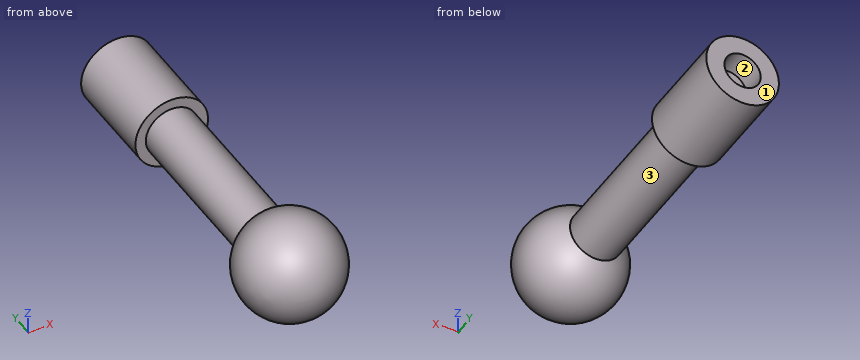
```python
from build123d import *

# Parameters (mm, degrees)
SKETCH3_W          = 7
SKETCH3_H          = 18.520312213
SKETCH4_R          = 3.5
CUT_EXTRUDE1_DEPTH = 5


with BuildPart() as part:
    # Sketch1 → Revolve1 (revolve)
    with BuildSketch(Plane.XY, mode=Mode.PRIVATE) as revolve1_sk:
        with BuildLine():
            Line((0, 41.73429327), (5, 41.73429327))
            Line((5, 41.73429327), (5, -8.26570673))
            ThreePointArc((5, -8.26570673), (9.659258263, -19.514151219), (0, -26.925960768))
            Line((0, -26.925960768), (0, 41.73429327))
        make_face()
    revolve(revolve1_sk.sketch.rotate(Axis((0, 41.73429327, 0), (0, -1, 0)), 180), axis=Axis((0, 41.73429327, 0), (0, -1, 0)))

    # Sketch3 → Revolve3 (revolve)
    with BuildSketch(Plane.XY, mode=Mode.PRIVATE) as revolve3_sk:
        with Locations((3.5, 32.474137164)):
            Rectangle(SKETCH3_W, SKETCH3_H)
    revolve(revolve3_sk.sketch.rotate(Axis((0, 41.73429327, 0), (0, -1, 0)), 90), axis=Axis((0, 41.73429327, 0), (0, -1, 0)))

    # Sketch4 → Cut-Extrude1 (cut)
    with BuildSketch(Plane(origin=(0, 41.73429327, 0), x_dir=(1, 0, 0), z_dir=(0, 1, 0))):
        with Locations(Location((0, 0, 0), (0, 0, 180))):
            Circle(SKETCH4_R)
    extrude(amount=-CUT_EXTRUDE1_DEPTH, mode=Mode.SUBTRACT)


solid = part.part
```
Read the model definition and answer for the solid it produces. Units are mm, in the model's axes. Face numbers are marked on the shaded views. Give positions to 0.01 mm unless a question says otherwise; leave off trailing zeros. Loops run counter-clockwise (first coordinate to the right, second up) from the corner with the lowest first, then second, coordinate; pieces in that order, holes last.
Item 1: The part is cut by section A-A (x = 0). Write down the section's boundary in (y, z).
Item 2: The mould has two halves that part along Z. Classify the marked faces 1, 2 and 3: released by +Z, released by -Z, zero draft, split by the parting line, or undercut.
Item 3: Find the intervals of material crossed by line 1 along Y through (x, z) = (-5.25, -0.75); line 2 along Z through (x, y) = (1.75, 28); line 3 along Z through (x, y) = (3.75, 15), in increasing order.
Item 4: The part is cut by section C-C (x = -6). Write down the section's boundary in (y, z), and give its area (3 significant figures).
Item 5: The part is cut by section B-B (z = 0). Write down the section's boundary in (x, y).
Item 6: Each of these flat-tipped pins is pushed along its axis until it touches: pin 1 Ø12 at (y, z) = (21.5, -1) entering from +X; pin 2 Ø8 at (y, z) = (6.5, 1) entering from +X; pin 3 Ø6.5 at (x, z) = (0, 0) entering from +Y; pin 4 Ø3 at (x, y) = (7, -6) entering from +Z. Where does it stop, or does it pass through?
Item 7: The part is cut by section D-D (y = 15.5). Write down the section's boundary in (x, z), and give its area (3 significant figures).
Taken from the geometry:
1. outline: (-8.27, -5) - (23.21, -5) - (23.21, -7) - (41.73, -7) - (41.73, -3.5) - (36.73, -3.5) - (36.73, 3.5) - (41.73, 3.5) - (41.73, 7) - (23.21, 7) - (23.21, 5) - (-8.27, 5) arc R10 ccw (long way) to start
2. face 1: zero draft
2. face 2: undercut
2. face 3: split by the parting line
3. line 1: y = -25.4 to -8.45, 23.21 to 41.73
3. line 2: z = -6.78 to 6.78
3. line 3: z = -3.31 to 3.31
4. outline: circle Ø16 at (-16.93, 0); (23.21, -3.61) - (41.73, -3.61) - (41.73, 3.61) - (23.21, 3.61) - close
4. area: 335 mm2
5. outline: (-7, 23.21) - (-5, 23.21) - (-5, -8.27) arc R10 ccw (long way) to (5, -8.27) - (5, 23.21) - (7, 23.21) - (7, 41.73) - (3.5, 41.73) - (3.5, 36.73) - (-3.5, 36.73) - (-3.5, 41.73) - (-7, 41.73) - close
6. pin 1: stops at x = 7
6. pin 2: stops at x = 5
6. pin 3: stops at y = 36.73
6. pin 4: passes through
7. outline: circle Ø10 at (0, 0)
7. area: 78.5 mm2
